Part model, mm, in its own coordinate system. A direction names the side the tool comes from. Give positions to 0.01 mm unless a question says otherwise; leave off trailing zeros. Order: outer loops, then holes, each group sorted by start corner. A loop starts at its lowest first (then second) coordinate and runs counter-clockwise, first axis right, second up. Notation, with made-up numbers: (74.5, 83) -> (121.5, 83) arc R16 cw to (121.5, 109) -> close; hole circle Ø8 at (61.5, 89). An arc over 180 degrees is marked (long way). Write item = value, one per line. Start each with the question number.
(1) Saw through at C-C, the plane y = -18. List the corners of the cut face in (x, z).
(2) Saw through at D-D, the plane y = 11. List the corners of the cut face in (x, z).
(3) Saw through at A-A, the plane z = 0. List the corners of the cut face in (x, y).
(4) Saw through at B-B, the plane x = 0. List the corners of the cut face in (y, z).
(5) Flat gauge pins, fed straight in: pin 1 (3 mm diameter, centred on y = -2, z = 4.5, fed in from +X); pin 2 (2 mm diameter, centred on y = 9, z = -6.5, fed in from +X); pin 3 (1 mm diameter, centred on y = -6.5, z = 8, fed in from +X); pin 4 (12 mm diameter, centred on x = -2.5, y = -14, fed in from -Z). Where does each tip first touch, or does it go through?
(6) Which spindle directions (+Z, -Z, +X, -X, +Y, -Y) get a long thin tool onto all of the face, cutting with end or side? Do faces 1 (the cylindrical face through (-1.5, -9.9, 11.4)), 2 (the flat face through (3, 0, -3)). Say none if no direction does.
(7) Probe line 1 along X through (y, z) = (-15.5, -8.5); line 2 along Y through (x, z) = (-5.5, -0.75); line 3 along X through (y, z) = (-10, -0.75). List the from-to ranges inside material, lowest first. Write a range as from..to.
from build123d import *

# Parameters (mm, degrees)
F0_R     = 11.5
F1_DEPTH = 20
F2_R     = 5
F3_R     = 3.910161
F4_DEPTH = 15
F5_SIZE  = 0.5


with BuildPart() as f1:
    # F0 (on Front) → F1 (new body)
    with BuildSketch(Plane.XZ):
        Circle(F0_R)
    extrude(amount=F1_DEPTH)

    # F2
    f2_edges = [f1.edges().sort_by_distance(p)[0] for p in [
        (-11.5, -20, 0),
        (-11.5, 0, 0),
    ]]
    fillet(f2_edges, radius=F2_R)

    # F3 (on Front) → F4 (join)
    with BuildSketch(Plane.XZ):
        Circle(F3_R)
    extrude(amount=-F4_DEPTH)

    # F5
    f5_edges = [f1.edges().sort_by_distance(p)[0] for p in [
        (-3.910161, 15, 0),
    ]]
    chamfer(f5_edges, length=F5_SIZE)


solid = f1.part
Results list:
q1.outline = circle Ø21 at (0, 0)
q2.outline = circle Ø7.82 at (0, 0)
q3.outline = (-11.5, -15) arc R5 ccw to (-6.5, -20) -> (6.5, -20) arc R5 ccw to (11.5, -15) -> (11.5, -5) arc R5 ccw to (6.5, 0) -> (3.91, 0) -> (3.91, 14.5) -> (3.41, 15) -> (-3.41, 15) -> (-3.91, 14.5) -> (-3.91, 0) -> (-6.5, 0) arc R5 ccw to (-11.5, -5) -> close
q4.outline = (-20, -6.5) arc R5 ccw to (-15, -11.5) -> (-5, -11.5) arc R5 ccw to (0, -6.5) -> (0, -3.91) -> (14.5, -3.91) -> (15, -3.41) -> (15, 3.41) -> (14.5, 3.91) -> (0, 3.91) -> (0, 6.5) arc R5 ccw to (-5, 11.5) -> (-15, 11.5) arc R5 ccw to (-20, 6.5) -> close
q5.pin_1 = 10.57
q5.pin_2 = through
q5.pin_3 = 8.72
q5.pin_4 = -11.5
q6.face_1 = +Y, -Y
q6.face_2 = +Y
q7.line_1 = -7.71..7.71
q7.line_2 = -20..0
q7.line_3 = -11.48..11.48
